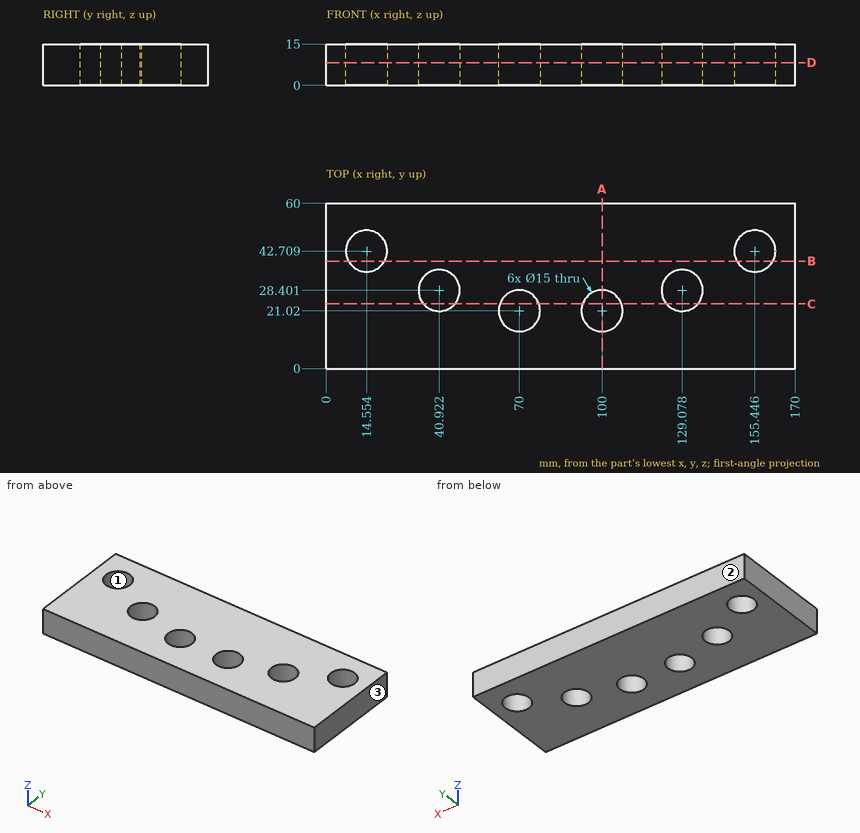
Job drawing, mm, ordinate dimensions from the low corner. One solid piece. Round coordinates to 2 decimals unless told otherwise and drop trailing zeros. Loops run counter-clockwise (first coordinate to the right, second up) from the corner with the lowest first, then second, coordinate; pieces in that order, holes last. Notation, with made-up numbers: M 26.5,-1 L 45.5,-1 A20 cw 45.5,19 Z; hole C 82,-22.5 d6. An arc over 180 degrees is marked long. One line per question, with ' | ' between items. Start each with the question number.
Item 1: Wall check: line 1 (X direction, y = 23, z = 1.25) (1 decimal); line 2 (X direction, y = 34.5, z = 5.5) (1 decimal); line 3 (X direction, y = 26.5, z = 13.75) (1 decimal). Give the ranges that are in metal, low to high.
Item 2: Cut at B-B, the plane y = 39. Write the cut outline in (x, z) (1 decimal), plus the area to 3 significant figures.
Item 3: Cut at C-C, the plane y = 23.5. Write the cut outline in (x, z) (1 decimal).
Item 4: Cut at D-D, the plane z = 8.25. Write the cut outline in (x, y).
Item 5: Two-plate mould, pull along X, no slides. Class the marked faces 1, 2 and 3: pulls with the +X half, pulls with the -X half, needs draft (parallel to the pull), parting line crosses it, or undercut.
Item 6: Cut at A-A, the plane x = 100. Write the cut outline in (y, z), plus the area to 3 significant figures.
Responses:
1) line 1: x = 0 to 35.7, 46.1 to 62.8, 77.2 to 92.8, 107.2 to 123.9, 134.3 to 170 | line 2: x = 0 to 36.6, 45.3 to 124.7, 133.4 to 170 | line 3: x = 0 to 33.7, 48.2 to 64.9, 75.1 to 94.9, 105.1 to 121.8, 136.3 to 170
2) outline: M 0,0 L 8,0 L 8,15 L 0,15 Z; M 21.1,0 L 148.9,0 L 148.9,15 L 21.1,15 Z; M 162,0 L 170,0 L 170,15 L 162,15 Z | area: 2,160 mm²
3) outline: M 0,0 L 35.2,0 L 35.2,15 L 0,15 Z; M 46.6,0 L 62.9,0 L 62.9,15 L 46.6,15 Z; M 77.1,0 L 92.9,0 L 92.9,15 L 77.1,15 Z; M 107.1,0 L 123.4,0 L 123.4,15 L 107.1,15 Z; M 134.8,0 L 170,0 L 170,15 L 134.8,15 Z
4) outline: M 0,0 L 170,0 L 170,60 L 0,60 Z; hole C 14.55,42.71 d15; hole C 40.92,28.4 d15; hole C 70,21.02 d15; hole C 100,21.02 d15; hole C 129.08,28.4 d15; hole C 155.45,42.71 d15
5) face 1: undercut | face 2: needs draft | face 3: pulls with the +X half
6) outline: M 0,0 L 13.52,0 L 13.52,15 L 0,15 Z; M 28.52,0 L 60,0 L 60,15 L 28.52,15 Z | area: 675 mm²
